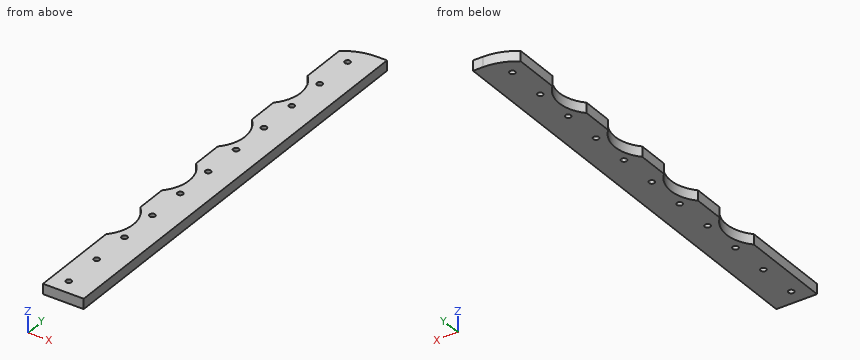
from build123d import *

# Parameters (mm, degrees)
SKETCH1_W           = 25.4
SKETCH1_H           = 276.225
BOSS_EXTRUDE1_DEPTH = 6.35
CUT_EXTRUDE1_DEPTH  = 7.35
SKETCH3_R           = 1.75
CUT_EXTRUDE2_DEPTH  = 7.35
LPATTERN1_COUNT     = 11
LPATTERN1_PITCH     = 25.4
SKETCH4_R           = 22.225
CUT_EXTRUDE3_DEPTH  = 7.35
LPATTERN2_COUNT     = 4
LPATTERN2_PITCH     = 50.8


with BuildPart() as part:
    # Sketch1 → Boss-Extrude1 (new body)
    with BuildSketch(Plane.XY):
        with Locations((-12.7, 138.1125)):
            Rectangle(SKETCH1_W, SKETCH1_H)
    extrude(amount=BOSS_EXTRUDE1_DEPTH)

    # Sketch2 → Cut-Extrude1 (cut, through all)
    with BuildSketch(Plane.XY.offset(6.35)):
        with BuildLine():
            Line((-6.35, 276.225), (-31.763279736, 276.225))
            Line((-31.763279736, 276.225), (-31.763279736, 263.507280815))
            ThreePointArc((-31.763279736, 263.507280815), (-20.55893353, 272.86811022), (-6.35, 276.225))
        make_face()
    extrude(amount=-CUT_EXTRUDE1_DEPTH, mode=Mode.SUBTRACT)

    # Sketch3 → Cut-Extrude2 (cut, through all)
    with BuildSketch(Plane.XY.offset(6.35)):
        with Locations((-15.875, 263.525)):
            Circle(SKETCH3_R)
    cut_extrude2 = extrude(amount=-CUT_EXTRUDE2_DEPTH, mode=Mode.SUBTRACT)

    # LPattern1: Cut-Extrude2 ×11
    with Locations(*[(0, -i * LPATTERN1_PITCH, 0) for i in range(1, LPATTERN1_COUNT)]):
        add(cut_extrude2, mode=Mode.SUBTRACT)

    # Sketch4 → Cut-Extrude3 (cut, through all)
    with BuildSketch(Plane.XY.offset(6.35)):
        with Locations((-41.275, 225.425)):
            Circle(SKETCH4_R)
    cut_extrude3 = extrude(amount=-CUT_EXTRUDE3_DEPTH, mode=Mode.SUBTRACT)

    # LPattern2: Cut-Extrude3 ×4
    with Locations(*[(0, -i * LPATTERN2_PITCH, 0) for i in range(1, LPATTERN2_COUNT)]):
        add(cut_extrude3, mode=Mode.SUBTRACT)


solid = part.part
Input: part model. Units: mm. Frame: model coordinates. Round coordinates to 2 decimals unless told otherwise and drop trailing zeros. Order: outer loops, then holes, each group sorted by start corner. A loop starts at its lowest first (then second) coordinate and runs counter-clockwise, first axis right, second up. Notation, with made-up numbers: (40, 87) - (60, 87) arc R19 cw to (60, 100) - close; hole circle Ø8 at (-30.5, 54). An arc over 180 degrees is marked (long way). Use a Markdown table: item, result.
1. Section B-B on y = 72. Return the cut outline in (x, z).
Evaluation:
| item | result |
|---|---|
| outline | (-19.07, 0) - (0, 0) - (0, 6.35) - (-19.07, 6.35) - close |
2. Section A-A on z = 4.5. State how many separate pieces and enclosed holes the cut face has, then the cut area to 3 significant figures.
Evaluation:
| item | result |
|---|---|
| separate pieces | 1 |
| enclosed holes | 11 |
| area | 6,330 mm^2 |
3. Material intervals for probe 1 along Y at (x, z) = (-22.75, 1); probe 2 along Y at (x, z) = (-21.5, 0.75); probe 3 along Y at (x, z) = (-7, 0.5), sorted ascending.
Evaluation:
| item | result |
|---|---|
| probe 1 | 0 to 60.75, 85.3 to 111.55, 136.1 to 162.35, 186.9 to 213.15, 237.7 to 271.66 |
| probe 2 | 0 to 62.88, 83.17 to 113.68, 133.97 to 164.48, 184.77 to 215.28, 235.57 to 272.38 |
| probe 3 | 0 to 276.22 |
4. First-contact query: pin 1 (3 mm diameter, centred on x = -15.875, y = 34.925, fed in from -Z); pin 2 (3 mm diameter, centred on x = -22, z = 2.5, fed in from +Y). Flat tips, straight axial feed; report the tip coordinate or a pass-through.
Evaluation:
| item | result |
|---|---|
| pin 1 | through |
| pin 2 | y = 272.9 |
